Could you check a few things on this model? Use its own coordinates, in mm. Coordinates: 2 decimals unless noted, no trailing zeros. Write each loop counter-clockwise with the first axis right and the second up, starting at its lowest first coordinate (ties: lowest second). Pieces come first, ordered by that corner, then holes. Notation, with made-up numbers: M -4,-12.75 L 23,-12.75 A15 cw 23,-2.75 Z; hole C -39,10 d8. An arc over 180 degrees is marked long. Answer as CSV lines item,"result". Start each with the question number.
Item 1: Suppose I cut it at B-B, the plane x = 15. Write out the boundary of the cut face in (y, z).
Item 2: Suppose I cut it at D-D, the plane x = 3.5. Write out the boundary of the cut face in (y, z).
Item 3: I'm going to push a flat-ended pin straight in: P1, Ø18, axis at x = 8.22, y = 36.01, coming from the -Z side (3 decimals). Where does the tip first touch, or does it pass through?
Item 4: We'd pull the mould along Y, two halves only. Please class faces 1 (the flat face through (8, 56.009, 1)), 2 (the flat face through (8, -43.991, 1)), 3 (the cylindrical face through (-7.109, 38.488, 1.521)): +Y half, -Y half, draft (parallel to the pull), parting line (faces both ways), or undercut.
Item 5: Suppose I cut it at C-C, the plane x = 23. Write out the boundary of the cut face in (y, z).
Item 6: If I drill on line 1 along Y through (x, z) = (-7, 0.85); line 2 along X through (y, z) = (36, 0.4); line 3 along Y through (x, z) = (23, 1.05), over which ranges is the centre line in solid material (lowest first)? Write a range as [from, to].
Item 7: Suppose I cut it at A-A, the plane z = 0.45. Write out the boundary of the cut face in (x, y).
```python
from build123d import *

# Parameters (mm, degrees)
SZKIC1_W                    = 50
SZKIC1_H                    = 100
SZKIC1_R                    = 2.5
DODANIE_WYCI_GNI_CIE1_DEPTH = 3
SZKIC2_R                    = 10
SZKIC2_R_2                  = 2.5
WYTNIJ_WYCI_GNI_CIE1_DEPTH  = 3


with BuildPart() as part:
    # Szkic1 → Dodanie-wyciągnięcie1 (new body)
    with BuildSketch(Plane.XY):
        with Locations((8.216170281, 6.009174312)):
            Rectangle(SZKIC1_W, SZKIC1_H)
        with Locations((23.216170281, -33.990825688)):
            Circle(SZKIC1_R, mode=Mode.SUBTRACT)
        with Locations((-6.783829719, -33.990825688)):
            Circle(SZKIC1_R, mode=Mode.SUBTRACT)
        with Locations((23.216170281, -14.524318973)):
            Circle(SZKIC1_R, mode=Mode.SUBTRACT)
        with Locations((-6.783829719, -13.990825688)):
            Circle(SZKIC1_R, mode=Mode.SUBTRACT)
    extrude(amount=DODANIE_WYCI_GNI_CIE1_DEPTH)

    # Szkic2 → Wytnij-wyciągnięcie1 (cut)
    with BuildSketch(Plane.XY.offset(3)):
        with Locations((8.216170281, 36.009174312)):
            Circle(SZKIC2_R)
        with Locations((-6.783829719, 36.009174312)):
            Circle(SZKIC2_R_2)
        with Locations((23.216170281, 36.009174312)):
            Circle(SZKIC2_R_2)
    extrude(amount=-WYTNIJ_WYCI_GNI_CIE1_DEPTH, mode=Mode.SUBTRACT)


solid = part.part
```
Ans:
1,outline,"M -43.99,0 L 28.66,0 L 28.66,3 L -43.99,3 Z; M 43.36,0 L 56.01,0 L 56.01,3 L 43.36,3 Z"
2,outline,"M -43.99,0 L 27.19,0 L 27.19,3 L -43.99,3 Z; M 44.83,0 L 56.01,0 L 56.01,3 L 44.83,3 Z"
3,P1,"passes through"
4,face 1,"+Y half"
4,face 2,"-Y half"
4,face 3,"undercut"
5,outline,"M -43.99,0 L -36.48,0 L -36.48,3 L -43.99,3 Z; M -31.5,0 L -17.01,0 L -17.01,3 L -31.5,3 Z; M -12.03,0 L 33.52,0 L 33.52,3 L -12.03,3 Z; M 38.5,0 L 56.01,0 L 56.01,3 L 38.5,3 Z"
6,line 1,"y = [-43.99, -36.48], [-31.5, -16.48], [-11.5, 33.52], [38.5, 56.01]"
6,line 2,"x = [-16.78, -9.28], [-4.28, -1.78], [18.22, 20.72], [25.72, 33.22]"
6,line 3,"y = [-43.99, -36.48], [-31.5, -17.01], [-12.03, 33.52], [38.5, 56.01]"
7,outline,"M -16.78,-43.99 L 33.22,-43.99 L 33.22,56.01 L -16.78,56.01 Z; hole C -6.78,-33.99 d5; hole C -6.78,-13.99 d5; hole C -6.78,36.01 d5; hole C 8.22,36.01 d20; hole C 23.22,-33.99 d5; hole C 23.22,-14.52 d5; hole C 23.22,36.01 d5"
